Check sheet for the modelled part. Datum: model origin and axes. Units: mm. Give positions to 0.01 mm unless a question says otherwise; leave off trailing zeros. Order: outer loops, then holes, each group sorted by start corner. A loop starts at its lowest first (then second) coordinate and runs counter-clockwise, first axis right, second up.
```python
from build123d import *

# Parameters (mm, degrees)
F1_DEPTH = 1300
F2_R     = 5
F3_DEPTH = 25


with BuildPart() as f1:
    # F0 (on Right) → F1 (new body)
    with BuildSketch(Plane.YZ):
        Polygon((-17.320508, -30), (17.320508, -30), (34.641016, 0), (17.320508, 30), (-17.320508, 30), (-34.641016, 0), align=None)
    extrude(amount=F1_DEPTH)

    # F2 (on face) → F3 (join)
    with BuildSketch(Plane.YZ.offset(1300)):
        Circle(F2_R)
    extrude(amount=F3_DEPTH)


solid = f1.part
```
(1) Cross-section at B-B on z = -18. Enter the section's corners in (x, y), then the cut area to 3 significant figures.
Response values:
outline: (0, -24.25) - (1300, -24.25) - (1300, 24.25) - (0, 24.25) - close
area: 63,000 mm2
(2) Material ranges on L1, parallel to X at y = 2, z = -23; L2, parallel to Y at x = 1141.5, z = -0.5; L3, parallel to Y at x = 638, z = -5.5, recorded low to high.
Response values:
L1: x = 0 to 1300
L2: y = -34.35 to 34.35
L3: y = -31.47 to 31.47
(3) Cross-section at A-A on x = 997.5. Enter the section's corners in (y, z), then the cut area to 3 significant figures.
Response values:
outline: (-34.64, 0) - (-17.32, -30) - (17.32, -30) - (34.64, 0) - (17.32, 30) - (-17.32, 30) - close
area: 3,120 mm2
(4) Gauge pin test, flat ends, axial feed: pin 1 Ø6 at (x, y) = (379, 21) entering from -Z; pin 2 Ø10 at (x, z) = (380.5, -0.5) entering from +Y; pin 3 Ø1 at (x, y) = (431, 27) entering from +Z. Record the tip position at first contact, or that the pin passes through.
Response values:
pin 1: stops at z = -28.82
pin 2: stops at y = 34.64
pin 3: stops at z = 14.1
